CAD build for the part. Positions are in the model's coordinates, mm. A direction names the side the tool comes from. Round coordinates to 2 decimals unless told otherwise and drop trailing zeros. Order: outer loops, then holes, each group sorted by start corner. A loop starts at its lowest first (then second) coordinate and runs counter-clockwise, first axis right, second up. Notation, with made-up numbers: (66.5, -29.5) - (97.5, -29.5) arc R11 ccw to (97.5, -10.5) - close; hole circle Ø6 at (43, 45). An arc over 180 degrees is marked (long way). Write item = value, one per line.
from build123d import *

# Parameters (mm, degrees)
EXTRUDE_1_DEPTH = 10
EXTRUDE_2_DEPTH = 1


with BuildPart() as part:
    # 草图1 → 凸台-拉伸1 (new body)
    with BuildSketch(Plane(origin=(0, 0, 0), x_dir=(1, 0, 0), z_dir=(0, 1, 0))):
        with BuildLine():
            Line((-32.5, 76), (32.5, 76))
            ThreePointArc((32.5, 76), (36.035533906, 74.535533906), (37.5, 71))
            Line((37.5, 71), (37.5, -71))
            ThreePointArc((37.5, -71), (36.035533906, -74.535533906), (32.5, -76))
            Line((32.5, -76), (-32.5, -76))
            ThreePointArc((-32.5, -76), (-36.035533906, -74.535533906), (-37.5, -71))
            Line((-37.5, -71), (-37.5, 71))
            ThreePointArc((-37.5, 71), (-36.035533906, 74.535533906), (-32.5, 76))
        make_face()
    extrude(amount=EXTRUDE_1_DEPTH)

    # 草图2 → 凸台-拉伸2 (add)
    with BuildSketch(Plane(origin=(0, 10, 0), x_dir=(1, 0, 0), z_dir=(0, 1, 0))):
        with BuildLine():
            Line((-29, 63), (-29, 42))
            ThreePointArc((-29, 42), (-22.5, 35.5), (-16, 42))
            Line((-16, 42), (-16, 63))
            ThreePointArc((-16, 63), (-22.5, 69.5), (-29, 63))
        make_face()
    extrude(amount=EXTRUDE_2_DEPTH)


solid = part.part
(1) Tool access for faces 1 (the cylindrical face through (-22.4, 10.5, -69.5)), 2 (the flat face through (-23, 11, -53)), 3 (the cylindrical face through (-22.6, 10.5, -35.5)): list every direction of +Z, -Z, +X, -X, +Y, -Y with a clear straight run to the whole face (end or side of a thin tool).
Solved:
face_1 = -Z, +Y
face_2 = +Z, -Z, +X, -X, +Y
face_3 = +Z, +Y
(2) Band-saw the part on B-B on z = -13. List the corners of the cut face in (x, y).
Solved:
outline = (-37.5, 0) - (37.5, 0) - (37.5, 10) - (-37.5, 10) - close
(3) Band-saw the part on C-C on x = 0.5. List the corners of the cut face in (y, z).
Solved:
outline = (0, -76) - (10, -76) - (10, 76) - (0, 76) - close
(4) Drop flat-ended pins along their axis: pin 1 (1.5 mm diameter, centred on x = 21, z = -22, fed in from +Y); pin 2 (0.8 mm diameter, centred on y = 10.5, z = -48.5, fed in from -X). Give the stop position or say it passes through.
Solved:
pin_1 = 10
pin_2 = -29
(5) Band-saw the part on A-A on x = -22.5. List the corners of the cut face in (y, z), plus the area to 3 significant figures.
Solved:
outline = (0, -76) - (10, -76) - (10, -69.5) - (11, -69.5) - (11, -35.5) - (10, -35.5) - (10, 76) - (0, 76) - close
area = 1,550 mm²
(6) Probe line 1 along Y through (x, z) = (30.5, 50); line 2 along Z through (x, y) = (-33, 6). List the from-to ranges inside material, lowest first.
Solved:
line_1 = 0 to 10
line_2 = -75.97 to 75.97
